Part model, mm, in its own coordinate system. Face numbers are marked on the shaded views. A direction names the side the tool comes from. Give positions to 0.01 mm unless a question says otherwise; leave off trailing zeros. Write each loop counter-clockwise with the first axis right and the second up, starting at its lowest first coordinate (ties: lowest second). Pieces come first, ordered by that corner, then holes. Notation, with made-up numbers: M -15.75,55.25 L 31.25,55.25 A31 cw 31.25,90.25 Z; hole C 69,53.5 d8. An arc over 180 degrees is marked long. Use a Markdown table: item, result. Add a question column.
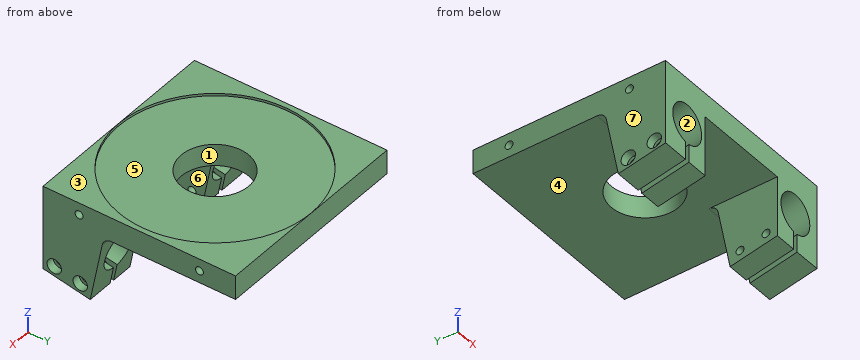
from build123d import *

# Parameters (mm, degrees)
SKETCH_1_W                  = 84
SKETCH_1_H                  = 80
SKETCH_1_R                  = 14
EXTRUDE_1_DEPTH             = 5
HOLE_WIZARD_M4_1_AT_2_COUNT = 2
HOLE_WIZARD_M4_1_AT_2_PITCH = 50
EXTRUDE_2_DEPTH             = 22
CUT_EXTRUDE_3_REACH         = 79
HOLE_START                  = -42
HOLE_WIZARD_2_OUTLINE_R     = 1.7
HOLE_WIZARD_2_DEPTH         = 11
HOLE_WIZARD_2_2_OUTLINE_R   = 3
HOLE_WIZARD_2_2_OUTLINE_R_2 = 1.7
HOLE_WIZARD_2_2_DEPTH       = 3.4
HOLE_WIZARD_M4_2_D          = 3.3
FILLET_1_R                  = 4
SKETCH_14_R                 = 39.95
CUT_EXTRUDE_6_DEPTH         = 1


# Read off the part's stored shape, not the designer's step: 打孔尺寸(%根据)内六角圆柱头螺钉的类型2
with BuildPart() as part:
    # 草图1 → 凸台-拉伸1 (new, symmetric)
    with BuildSketch(Plane.XY):
        Rectangle(SKETCH_1_W, SKETCH_1_H)
        Circle(SKETCH_1_R, mode=Mode.SUBTRACT)
    extrude(amount=EXTRUDE_1_DEPTH, both=True)

    # 草图4 → M4 螺纹孔1 (revolve, cut)
    with BuildSketch(Plane(origin=(-42, 25, 0), x_dir=(0, 0, 1), z_dir=(0, 1, 0))):
        Polygon((0, 0), (0, 14.491420021), (1.65, 13.5), (1.65, 0), align=None)
    hole_wizard_m4_1 = revolve(axis=Axis((-48.35, 25, 0), (1, 0, 0)), mode=Mode.SUBTRACT)

    # M4 螺纹孔1 at 2: M4 螺纹孔1 ×2
    with Locations(*[(0, -i * HOLE_WIZARD_M4_1_AT_2_PITCH, 0) for i in range(1, HOLE_WIZARD_M4_1_AT_2_COUNT)]):
        add(hole_wizard_m4_1, mode=Mode.SUBTRACT)

    # 草图6 → 凸台-拉伸2 (add)
    with BuildSketch(Plane.ZY.offset(42)):
        Polygon((-5, -14.766158372), (-5, -40), (-30, -40), (-33.816179908, -20.367456331), align=None)
    extrude_2 = extrude(amount=-EXTRUDE_2_DEPTH)

    # 切除-拉伸3: up to this plane
    cut_extrude_3_end = Plane(origin=(-42, -40, 5), z_dir=(0, 1, 0))
    # 草图7 → 切除-拉伸3 (cut, up to the surface)
    with BuildSketch(Plane(origin=(0, -13.292034521, 2.583709779), x_dir=(1, 0, 0), z_dir=(0, 0.9816271834476648, -0.19080899537654153)), mode=Mode.PRIVATE) as cut_extrude_3_sk1:
        with BuildLine():
            Line((-31, 37.081175318), (-29, 37.081175318))
            Line((-29, 37.081175318), (-29, 29.662905695))
            ThreePointArc((-29, 29.662905695), (-30, 13.725651762), (-31, 29.662905695))
            Line((-31, 29.662905695), (-31, 37.081175318))
        make_face()
    cut_extrude_3_tool1 = split(extrude(cut_extrude_3_sk1.sketch, amount=-CUT_EXTRUDE_3_REACH, mode=Mode.PRIVATE), bisect_by=cut_extrude_3_end, keep=Keep.BOTH, mode=Mode.PRIVATE)
    cut_extrude_3 = cut_extrude_3_tool1.solids().sort_by_distance((-30, -17.589666, -19.525688))[0]
    add(cut_extrude_3, mode=Mode.SUBTRACT)

    # 打孔尺寸(%根据)内六角圆柱头螺钉的类型2 outline → 打孔尺寸(%根据)内六角圆柱头螺钉的类型2 (cut)
    with BuildSketch(Plane.YZ.offset(HOLE_START)):
        with Locations((-35.310255285, -26.836727248)):
            Circle(HOLE_WIZARD_2_OUTLINE_R)
        with Locations((-24.512356267, -28.935626197)):
            Circle(HOLE_WIZARD_2_OUTLINE_R)
    hole_wizard_2 = extrude(amount=HOLE_WIZARD_2_DEPTH, mode=Mode.SUBTRACT)

    # Hole Wizard 2 2 outline → Hole Wizard 2 2 (cut)
    # profile 1 of 2: a face of its own
    with BuildSketch(Plane.YZ.offset(HOLE_START)):
        with Locations((-35.310255285, -26.836727248)):
            Circle(HOLE_WIZARD_2_2_OUTLINE_R)
        with Locations((-35.310255285, -26.836727248)):
            Circle(HOLE_WIZARD_2_2_OUTLINE_R_2, mode=Mode.SUBTRACT)
    # profile 2 of 2: a face of its own
    with BuildSketch(Plane.YZ.offset(HOLE_START)):
        with Locations((-24.512356267, -28.935626197)):
            Circle(HOLE_WIZARD_2_2_OUTLINE_R)
        with Locations((-24.512356267, -28.935626197)):
            Circle(HOLE_WIZARD_2_2_OUTLINE_R_2, mode=Mode.SUBTRACT)
    hole_wizard_2_2 = extrude(amount=HOLE_WIZARD_2_2_DEPTH, mode=Mode.SUBTRACT)

    # M4 螺纹孔2 (through all)
    with Locations(Plane(origin=(-20, 0, 0), x_dir=(0, 0, -1), z_dir=(1, 0, 0))):
        with Locations((28.935626197, -24.512356267), (26.836727248, -35.310255285)):
            hole_wizard_m4_2 = Hole(HOLE_WIZARD_M4_2_D / 2)

    # 镜向1: M4 螺纹孔1, 凸台-拉伸2, 切除-拉伸3, 打孔尺寸(%根据)内六角圆柱头螺钉的类型2, Hole Wizard 2 2, M4 螺纹孔2 across plane
    add(hole_wizard_m4_1.mirror(Plane(origin=(0, 0, 0), x_dir=(0, 0, 1), z_dir=(1, 0, 0))), mode=Mode.SUBTRACT)
    add(extrude_2.mirror(Plane(origin=(0, 0, 0), x_dir=(0, 0, 1), z_dir=(1, 0, 0))))
    add(cut_extrude_3.mirror(Plane(origin=(0, 0, 0), x_dir=(0, 0, 1), z_dir=(1, 0, 0))), mode=Mode.SUBTRACT)
    add(hole_wizard_2.mirror(Plane(origin=(0, 0, 0), x_dir=(0, 0, 1), z_dir=(1, 0, 0))), mode=Mode.SUBTRACT)
    add(hole_wizard_2_2.mirror(Plane(origin=(0, 0, 0), x_dir=(0, 0, 1), z_dir=(1, 0, 0))), mode=Mode.SUBTRACT)
    add(hole_wizard_m4_2.mirror(Plane(origin=(0, 0, 0), x_dir=(0, 0, 1), z_dir=(1, 0, 0))), mode=Mode.SUBTRACT)

    # 镜向1 copy 1 sketch → 镜向1 copy 1 (revolve, cut)
    with BuildSketch(Plane(origin=(42, -25, 0), x_dir=(0, 0, 1), z_dir=(0, 1, 0))):
        Polygon((0, 0), (0, -14.491420021), (1.65, -13.5), (1.65, 0), align=None)
    revolve(axis=Axis((48.35, -25, 0), (1, 0, 0)), mode=Mode.SUBTRACT)

    # 圆角1
    fillet_1_edges = [part.edges().sort_by_distance(p)[0] for p in [
        (-31, -14.766158372, -5),
        (31, -14.766158372, -5),
    ]]
    fillet(fillet_1_edges, radius=FILLET_1_R)

    # 草图14 → 切除-拉伸6 (cut)
    with BuildSketch(Plane.XY.offset(5)):
        Circle(SKETCH_14_R)
    extrude(amount=-CUT_EXTRUDE_6_DEPTH, mode=Mode.SUBTRACT)


solid = part.part
1. Cut at D-D (z = -21). Give the number of separate pieces and of enclosed holes in the cut face, then the cut area to 3 significant figures.
2. Tool access for the marked faces 4, 5, 6 and 7: list every direction of +Z, -Z, +X, -X, +Y, -Y with a clear straight run to the whole face (end or side of a thin tool).
3. Cut at C-C (y = 32.5). Write the cut outline in (x, z).
4. Drill centre lines: probe 1 along Y at (x, z) = (-34.25, 0); probe 2 along X at (y, z) = (-36, -15); probe 3 along X at (y, z) = (0, -1.75). Where is each one in solid material? Low to high. Write a range as [from, to].
5. Cut at B-B (y = 2.5). Write the cut outline in (x, z), then the cut area to 3 significant figures.
6. Mould opens along Z. For the marked faces 1, 2 and 3 say: released by +Z, released by -Z, zero draft, split by the parting line, or undercut.
7. Flat gauge pins, fed straight in: pin 1 (24 mm diameter, centred on x = 5, y = -16.5, fed in from -Z); pin 2 (5.5 mm diameter, centred on y = -24.51, z = -28.94, fed in from -X); pin 3 (2.5 mm diameter, centred on y = -24.51, z = -28.94, fed in from +X); pin 4 (5.5 mm diameter, centred on y = -24.51, z = -28.94, fed in from +X). Where does each tip first touch, or does it go through?
8. Cut at A-A (x = 0). Write the cut outline in (y, z).
A:
| question | item | result |
|---|---|---|
| 1 | separate pieces | 4 |
| 1 | enclosed holes | 0 |
| 1 | area | 398 mm² |
| 2 | face 4 | -Z, +Y |
| 2 | face 5 | +Z |
| 2 | face 6 | -Z, +Y, -Y |
| 2 | face 7 | +Z, -Z, -X, +Y, -Y |
| 3 | outline | M -42,-5 L 42,-5 L 42,5 L 23.23,5 L 23.23,4 L -23.23,4 L -23.23,5 L -42,5 Z |
| 4 | probe 1 | y = [-40, -26.65], [-23.35, 23.35], [26.65, 40] |
| 4 | probe 2 | x = [-42, -38], [-22, -20], [20, 22], [38, 42] |
| 4 | probe 3 | x = [-42, -14], [14, 42] |
| 5 | outline | M -42,-5 L -13.77,-5 L -13.77,4 L -39.87,4 L -39.87,5 L -42,5 Z; M 13.77,-5 L 42,-5 L 42,5 L 39.87,5 L 39.87,4 L 13.77,4 Z |
| 5 | area | 512 mm² |
| 6 | face 1 | zero draft |
| 6 | face 2 | undercut |
| 6 | face 3 | released by +Z |
| 7 | pin 1 | stops at z = -5 |
| 7 | pin 2 | stops at x = -38.6 |
| 7 | pin 3 | passes through |
| 7 | pin 4 | stops at x = 38.6 |
| 8 | outline | M -40,-5 L -14,-5 L -14,4 L -39.95,4 L -39.95,5 L -40,5 Z; M 14,-5 L 40,-5 L 40,5 L 39.95,5 L 39.95,4 L 14,4 Z |
